```python
from build123d import *

# Parameters (mm, degrees)
F0_R          = 70.553851
F1_DEPTH      = 25.4
F2_R          = 18.763513
F3_DEPTH      = 61.607625
F4_R          = 10.074339
F5_DEPTH      = 81.966516
F5_DEPTH_BACK = 109.91749


with BuildPart() as f1:
    # F0 (on Front) → F1 (new body)
    with BuildSketch(Plane.XZ):
        Circle(F0_R)
    extrude(amount=F1_DEPTH)

    # F2 (on face) → F3 (cut)
    with BuildSketch(Plane.XZ.offset(25.4)):
        with Locations((0, 37.898846)):
            Circle(F2_R)
    extrude(amount=-F3_DEPTH, mode=Mode.SUBTRACT)

    # F4 (on face) → F5 (join, two sides)
    with BuildSketch(Plane.XZ.offset(25.4)) as f5_sk:
        Circle(F4_R)
    extrude(amount=F5_DEPTH)
    extrude(f5_sk.sketch, amount=-F5_DEPTH_BACK)


solid = f1.part
```
Input: part model. Units: mm. Frame: model coordinates. A direction names the side the tool comes from. Round coordinates to 2 decimals unless told otherwise and drop trailing zeros. Order: outer loops, then holes, each group sorted by start corner. A loop starts at its lowest first (then second) coordinate and runs counter-clockwise, first axis right, second up. Notation, with made-up numbers: (22, -14) - (77, -14) arc R27 ccw to (77, 16) - close; hole circle Ø6 at (59, 23). An arc over 180 degrees is marked (long way). Answer in a Markdown table with one row per item.
Item 1: Mould query, pull axis Z, two halves, no side actions, for faces 4 (the flat face through (0, 84.517, 0)), 5 (the cylindrical face through (-4.068, -12.878, 19.582)), 6 (the cylindrical face through (-15.295, -12.522, -68.876)). Classes: released by +Z, released by -Z, zero draft, split by the parting line, or undercut.
Model answer:
| item | result |
|---|---|
| face 4 | zero draft |
| face 5 | undercut |
| face 6 | split by the parting line |
Item 2: Section query A-A (x = 0). Return the cut outline in (y, z), then the cut area to 3 significant figures.
Model answer:
| item | result |
|---|---|
| outline | (-107.37, -10.07) - (-25.4, -10.07) - (-25.4, -70.55) - (0, -70.55) - (0, -10.07) - (84.52, -10.07) - (84.52, 10.07) - (0, 10.07) - (0, 19.14) - (-25.4, 19.14) - (-25.4, 10.07) - (-107.37, 10.07) - close; (-25.4, 56.66) - (0, 56.66) - (0, 70.55) - (-25.4, 70.55) - close |
| area | 5,990 mm² |
Item 3: Reachability of faces 1 (the flat face through (0, -107.367, 0)), 2 (the cylindrical face through (-7.995, -65.809, -6.13)), 3 (the cylindrical face through (-7.995, 41.667, -6.13)) from +Z, -Z, +X, -X, +Y, -Y: full face, straight path, thin tool, end or side. Return the list, or none.
Model answer:
| item | result |
|---|---|
| face 1 | +Z, -Z, +X, -X, -Y |
| face 2 | -Y |
| face 3 | +Y |
Item 4: Section query B-B (z = 0). Return the cut outline in (x, y), then the cut area to 3 significant figures.
Model answer:
| item | result |
|---|---|
| outline | (-70.55, -25.4) - (-10.07, -25.4) - (-10.07, -107.37) - (10.07, -107.37) - (10.07, -25.4) - (70.55, -25.4) - (70.55, 0) - (10.07, 0) - (10.07, 84.52) - (-10.07, 84.52) - (-10.07, 0) - (-70.55, 0) - close |
| area | 6,940 mm² |
Item 5: Line query: line 1 (Z direction, x = 0, y = -19); line 2 (Y direction, x = -40.5, z = 52); line 3 (X direction, y = -9.5, z = 26). Output: solid intervals per line, ascending.
Model answer:
| item | result |
|---|---|
| line 1 | z = -70.55 to 19.14, 56.66 to 70.55 |
| line 2 | y = -25.4 to 0 |
| line 3 | x = -65.59 to -14.51, 14.51 to 65.59 |
Item 6: Section query C-C (z = 42). Return the cut outline in (x, y).
Model answer:
| item | result |
|---|---|
| outline | (-56.69, -25.4) - (-18.31, -25.4) - (-18.31, 0) - (-56.69, 0) - close; (18.31, -25.4) - (56.69, -25.4) - (56.69, 0) - (18.31, 0) - close |
Item 7: Pin query (flat end, axial travel): pin 1 (4 mm diameter, centred on x = 22.5, z = -42, fed in from +Y); pin 2 (8 mm diameter, centred on x = 2, y = -40, fed in from +Z); pin 3 (5 mm diameter, centred on x = -54.5, z = -33, fed in from -Y); pin 4 (5 mm diameter, centred on x = -15, y = 9, fed in from +Z). Return the tip coordinate at first contact, or that it passes through.
Model answer:
| item | result |
|---|---|
| pin 1 | stops at y = 0 |
| pin 2 | stops at z = 10.07 |
| pin 3 | stops at y = -25.4 |
| pin 4 | passes through |
Item 8: Section query D-D (y = 54.5). Return the cut outline in (x, z).
Model answer:
| item | result |
|---|---|
| outline | circle Ø20.15 at (0, 0) |
